Check sheet for the modelled part. Datum: model origin and axes. Units: mm. Coordinates: 2 decimals unless noted, no trailing zeros. Loops run counter-clockwise (first coordinate to the right, second up) from the corner with the lowest first, then second, coordinate; pieces in that order, holes last. Notation, with made-up numbers: (14.5, 65.25) - (49.5, 65.25) arc R27 cw to (49.5, 100.25) - close; hole circle Ø4 at (30, 78.5). An arc over 180 degrees is marked (long way). Use a Markdown table: item, result. Add a question column.
1) Thickness scan on line 1 (Z direction, x = 70, y = 2.2); line 2 (X direction, y = 2.85, z = 7.5); line 3 (X direction, y = 2.15, z = 20). Record the ranges inside material, lowest first.
2) Sectioned sample at A-A, the plane x = 70. Enter the section's corners in (y, z) (3 decimals), then the cut area to 3 significant figures.
3) Sectioned sample at C-C, the plane y = 1. State how many separate pieces and enclosed holes the cut face has, then the cut area to 3 significant figures.
4) Sectioned sample at D-D, the plane z = 29.5. Enter the section's corners in (x, y) (3 decimals), then the cut area to 3 significant figures.
5) Sectioned sample at B-B, the plane z = 3.5. Enter the section's corners in (x, y) (3 decimals), then the cut area to 3 significant figures.
from build123d import *

# Parameters (mm, degrees)
SKETCH1_R           = 11.15
SKETCH1_R_2         = 7.5
SKETCH1_R_3         = 3.325
BOSS_EXTRUDE1_DEPTH = 3.175


with BuildPart() as part:
    # Sketch1 → Boss-Extrude1 (new body)
    with BuildSketch(Plane(origin=(0, 0, 0), x_dir=(1, 0, 0), z_dir=(0, 1, 0))):
        with BuildLine():
            ThreePointArc((-126.258214395, 35), (-161.258214395, 0), (-126.258214395, -35))
            Line((-126.258214395, -35), (246.658214395, -35))
            Line((246.658214395, -35), (246.658214395, 35))
            Line((246.658214395, 35), (-126.258214395, 35))
        make_face()
        with Locations((-126.258214395, 0)):
            Circle(SKETCH1_R, mode=Mode.SUBTRACT)
        with Locations((-70, -17.5)):
            Circle(SKETCH1_R_2, mode=Mode.SUBTRACT)
        with BuildLine():
            ThreePointArc((15, 0), (0, -15), (-15, 0))
            ThreePointArc((-15, 0), (0, 15), (15, 0))
        make_face(mode=Mode.SUBTRACT)
        with Locations((70, -17.5)):
            Circle(SKETCH1_R_2, mode=Mode.SUBTRACT)
        with Locations((173.958214395, -20)):
            Circle(SKETCH1_R_3, mode=Mode.SUBTRACT)
        with Locations((233.958214395, -20)):
            Circle(SKETCH1_R_3, mode=Mode.SUBTRACT)
        with Locations((-70, 17.5)):
            Circle(SKETCH1_R_2, mode=Mode.SUBTRACT)
        with Locations((126.258214395, 0)):
            Circle(SKETCH1_R, mode=Mode.SUBTRACT)
        with Locations((70, 17.5)):
            Circle(SKETCH1_R_2, mode=Mode.SUBTRACT)
        with Locations((173.958214395, 20)):
            Circle(SKETCH1_R_3, mode=Mode.SUBTRACT)
        with Locations((233.958214395, 20)):
            Circle(SKETCH1_R_3, mode=Mode.SUBTRACT)
    extrude(amount=BOSS_EXTRUDE1_DEPTH)


solid = part.part
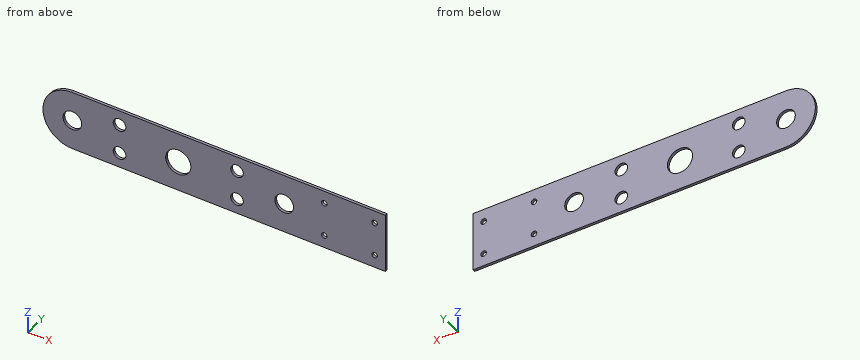
Solved:
| question | item | result |
|---|---|---|
| 1 | line 1 | z = -35 to -25, -10 to 10, 25 to 35 |
| 1 | line 2 | x = -160.45 to -134.51, -118.01 to -12.99, 12.99 to 118.01, 134.51 to 246.66 |
| 1 | line 3 | x = -154.98 to -77.07, -62.93 to 62.93, 77.07 to 170.63, 177.28 to 230.63, 237.28 to 246.66 |
| 2 | outline | (0, -35) - (3.175, -35) - (3.175, -25) - (0, -25) - close; (0, -10) - (3.175, -10) - (3.175, 10) - (0, 10) - close; (0, 25) - (3.175, 25) - (3.175, 35) - (0, 35) - close |
| 2 | area | 127 mm2 |
| 3 | separate pieces | 1 |
| 3 | enclosed holes | 11 |
| 3 | area | 25,700 mm2 |
| 4 | outline | (-145.093, 0) - (246.658, 0) - (246.658, 3.175) - (-145.093, 3.175) - close |
| 4 | area | 1,240 mm2 |
| 5 | outline | (-161.083, 0) - (-136.845, 0) - (-136.845, 3.175) - (-161.083, 3.175) - close; (-115.672, 0) - (-14.586, 0) - (-14.586, 3.175) - (-115.672, 3.175) - close; (14.586, 0) - (115.672, 0) - (115.672, 3.175) - (14.586, 3.175) - close; (136.845, 0) - (246.658, 0) - (246.658, 3.175) - (136.845, 3.175) - close |
| 5 | area | 1,070 mm2 |
